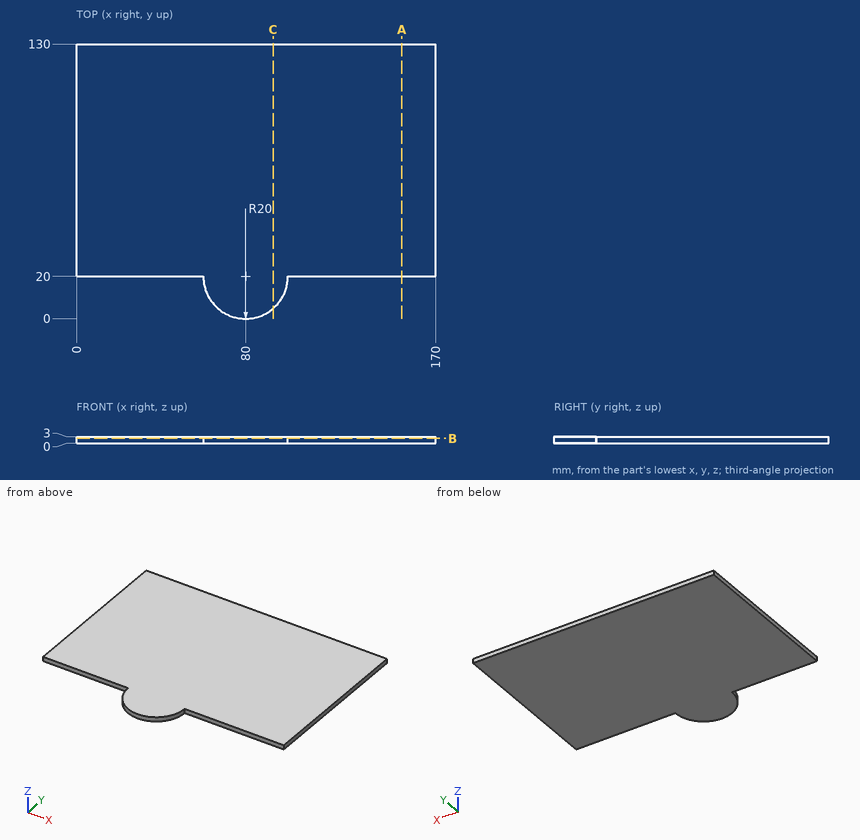
Study the drawing (mm; zero at the part's minimum x, y, z) and answer. Give positions to 0.01 mm unless a question says otherwise; leave off trailing zeros. Order: outer loops, then holes, each group sorted by start corner. A loop starts at its lowest first (then second) coordinate and runs counter-clockwise, first axis right, second up. Notation, with made-up numbers: (25.5, 16) -> (33.5, 16) arc R27 ccw to (33.5, 34) -> close; hole circle Ø2 at (-17, 29.25). An arc over 180 degrees is marked (long way). Write item = value, one per line.
1. Straight lines are drawn through the part: line 1 along Y through (x, z) = (162, 1.2); line 2 along X through (y, z) = (7.5, 1.4); line 3 along Y through (x, z) = (66.5, 1.35). For each, find the intervals that lie inside material, in ascending order.
Numbers:
line_1 = 20 to 130
line_2 = 64.39 to 95.61
line_3 = 5.24 to 130
2. A cutting plane is placed at C-C, the plane x = 93. Write down the section's boundary in (y, z).
Numbers:
outline = (4.8, 0) -> (130, 0) -> (130, 3) -> (4.8, 3) -> close
3. A cutting plane is placed at B-B, the plane z = 2.25. Write down the section's boundary in (x, y).
Numbers:
outline = (0, 20) -> (60, 20) arc R20 ccw to (100, 20) -> (170, 20) -> (170, 130) -> (0, 130) -> close
4. A cutting plane is placed at A-A, the plane x = 154. Write down the section's boundary in (y, z).
Numbers:
outline = (20, 0) -> (130, 0) -> (130, 3) -> (20, 3) -> close
5. Given pin 1 (1.5 mm diameter, centred on x = 127.5, z = 1, fed in from -Y), flat-ended and moving along its own axis, determine where the tip first touches the part or whether it passes through.
Numbers:
pin_1 = 20
